```python
from build123d import *

# Parameters (mm, degrees)
CROQUIS1_W  = 38
CROQUIS1_H  = 2.5
REDONDEO1_R = 0.25


with BuildPart() as part:
    # Croquis1 → Revolución1 (revolve)
    with BuildSketch(Plane.XY):
        with Locations((19, 1.25)):
            Rectangle(CROQUIS1_W, CROQUIS1_H)
    revolve(axis=Axis((0, 0, 0), (1, 0, 0)))

    # Redondeo1
    redondeo1_edges = [part.edges().sort_by_distance(p)[0] for p in [
        (38, -2.5, 0),
    ]]
    fillet(redondeo1_edges, radius=REDONDEO1_R)

    # Croquis3 → Cortar-Revolución1 (revolve, cut)
    with BuildSketch(Plane.XY):
        Polygon((38, 0), (37.5, 0), (38, 1), align=None)
    revolve(axis=Axis((38, 0, 0), (-1, 0, 0)), mode=Mode.SUBTRACT)


solid = part.part
```
Check sheet for the modelled part. Datum: model origin and axes. Units: mm. Give positions to 0.01 mm unless a question says otherwise; leave off trailing zeros. Loops run counter-clockwise (first coordinate to the right, second up) from the corner with the lowest first, then second, coordinate; pieces in that order, holes last. Notation, with made-up numbers: M 33,9 L 69,9 A11 cw 69,29 Z; hole C 89,63.25 d8. An arc over 180 degrees is marked long. Answer as CSV lines item,"result".
Item 1: Draft check along Y on faces 1 (the face through (37.53, -0.01, 0.06)), 2 (the face through (38, 1, -1)), 3 (the face through (19.14, -0.54, -2.44)). Enter one of: pulls with the +Y half, pulls with the -Y half, needs draft (parallel to the pull), parting line crosses it, or undercut.
Reply:
face 1,"undercut"
face 2,"needs draft"
face 3,"parting line crosses it"
Item 2: Scan lines: L1, parallel to Y at x = 30, z = -0.2; L2, parallel to Y at x = 34.5, z = 1.1 (3 decimals); L3, parallel to Z at x = 26, y = 1. Record each from-to range of solid material in increasing order.
Reply:
L1,"-2.49 to 2.49"
L2,"-2.245 to 2.245"
L3,"-2.29 to 2.29"
Item 3: Sectioned sample at A-A, the plane x = 27. Enter the section's corners in (y, z), then the cut area to 3 significant figures.
Reply:
outline,"C 0,0 d5"
area,"19.6 mm^2"
Item 4: Depth check by flat-ended pin: pin 1 Ø1 at (x, z) = (28.5, 1) entering from +Y. Enter the tip coordinate at first touch or a pass-through.
Reply:
pin 1,"y = 2.45"
